Source: three-view drawing plus pictorial views. Frame: mm from the lowest corner of the part. Round coordinates to 2 decimals unless told otherwise and drop trailing zeros. Write each loop counter-clockwise with the first axis right and the second up, starting at its lowest first coordinate (ties: lowest second). Pieces come first, ordered by that corner, then holes. Notation, with made-up numbers: (55.5, 88) - (104.5, 88) arc R13 cw to (104.5, 108) - close; hole circle Ø2 at (83.25, -37.75). An arc over 180 degrees is marked (long way). Write each question's results on one line, items separated by ' | '.
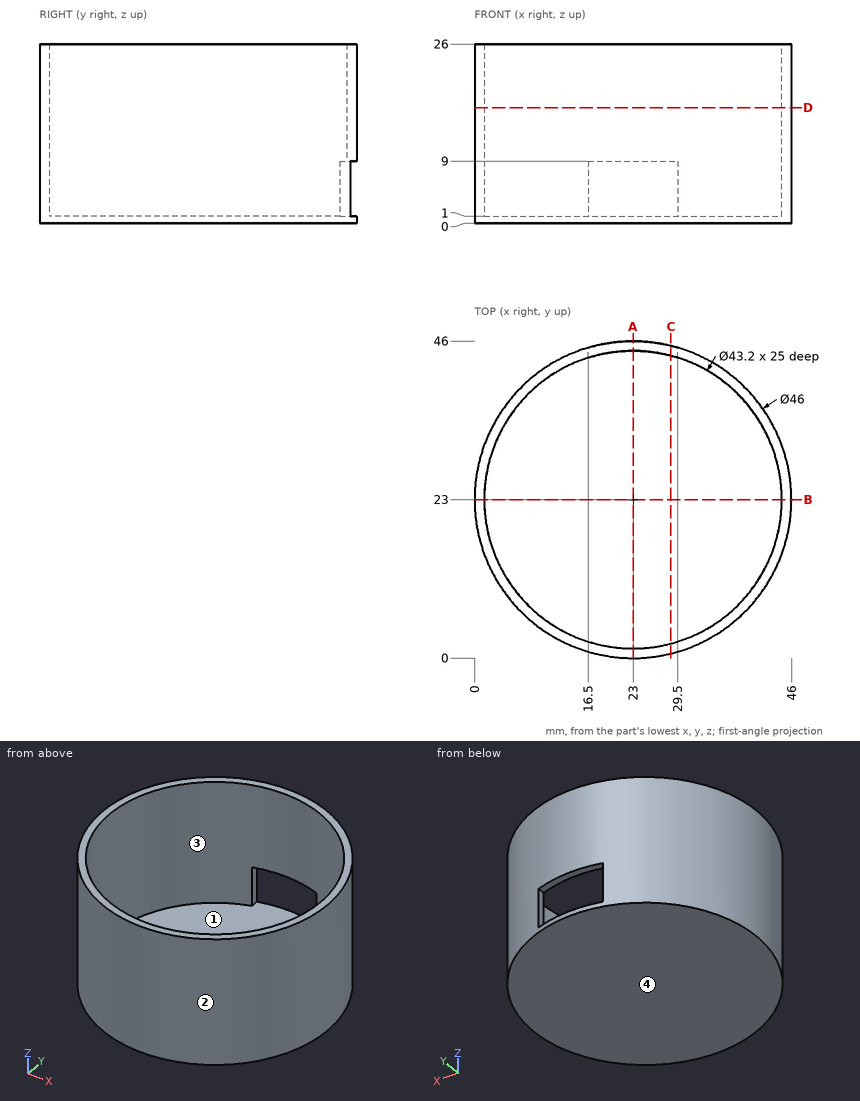
Q1. Section query B-B, the plane y = 23. Return loops of the section in (x, z), plus the area to 3 significant figures.
Answer block:
outline: (0, 0) - (46, 0) - (46, 26) - (44.6, 26) - (44.6, 1) - (1.4, 1) - (1.4, 26) - (0, 26) - close | area: 116 mm2
Q2. Ray query, line 1 along Y through (x, z) = (23, 20.75); line 2 along Y through (x, z) = (12.5, 18); line 3 along Y through (x, z) = (23, 7.5). Return the intervals inside material, ascending.
Answer block:
line 1: 0 to 1.4, 44.6 to 46 | line 2: 2.54 to 4.12, 41.88 to 43.46 | line 3: 0 to 1.4
Q3. Pin query (flat end, axial travel): pin 1 (8 mm diameter, centred on x = 32.5, z = 9.5, fed in from +Y); pin 2 (3 mm diameter, centred on x = 18, z = 21.5, fed in from +Y); pin 3 (0.7 mm diameter, centred on y = 44.5, z = 4, fed in from +X). Return the tip coordinate at first contact, or that it passes through.
Answer block:
pin 1: y = 45.33 | pin 2: y = 45.73 | pin 3: x = 32.04
Q4. Section query A-A, the plane x = 23. Return loops of the section in (y, z).
Answer block:
outline: (0, 0) - (46, 0) - (46, 1) - (1.4, 1) - (1.4, 26) - (0, 26) - close; (44.6, 9) - (46, 9) - (46, 26) - (44.6, 26) - close
Q5. Section query D-D, the plane z = 16.75. Return loops of the section in (x, y).
Answer block:
outline: circle Ø46 at (23, 23); hole circle Ø43.2 at (23, 23)
Q6. Section query C-C, the plane x = 28.5. Return loops of the section in (y, z).
Answer block:
outline: (0.67, 0) - (45.33, 0) - (45.33, 1) - (2.11, 1) - (2.11, 26) - (0.67, 26) - close; (43.89, 9) - (45.33, 9) - (45.33, 26) - (43.89, 26) - close
Q7. Mould query, pull axis Y, two halves, no side actions, for the marked faces 1, 2, 3 and 4. Classes: pulls with the +Y half, pulls with the -Y half, needs draft (parallel to the pull), parting line crosses it, or undercut.
Answer block:
face 1: undercut | face 2: parting line crosses it | face 3: undercut | face 4: needs draft
